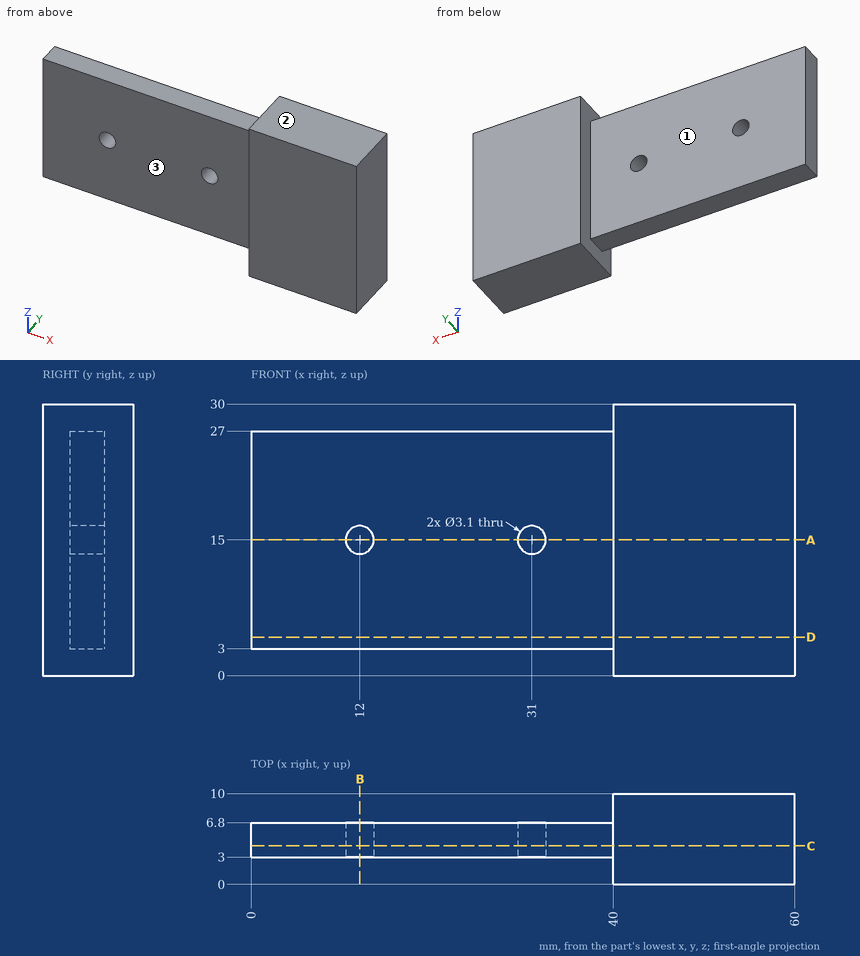
Geometry: see drawing. Coordinates: mm, zero at the bounding-box minimum. Round coordinates to 2 decimals unless told otherwise and drop trailing zeros. Write each loop counter-clockwise with the first axis right and the second up, starting at its lowest first coordinate (ties: lowest second). Pieces come first, ordered by that corner, then holes.
Item 1: Section query A-A (z = 15). Return loops of the section in (x, y), plus the area to 3 significant figures.
Item 2: Pin query (flat end, axial travel): P1, Ø1.9, axis at x = 12, z = 15, coming from the +Y side; P2, Ø3, axis at x = 21.5, z = 25.5, coming from the -Y side; P3, Ø6, axis at x = 32.5, y = 8, coming from the +Z side; P4, Ø4, axis at x = 17, y = 1.5, coming from the -Z side. Return the tip coordinate at first contact, or that it passes through.
Item 3: Material intervals for L1, parallel to X at y = 4.9, z = 15; L2, parallel to Z at x = 15, y = 5.25; L3, parallel to Y at x = 21.5, z = 21.25, sorted ascending.
Item 4: Section query B-B (x = 12). Return loops of the section in (y, z).
Item 5: Mould query, pull axis Y, two halves, no side actions, for the marked faces 1, 2 and 3. Classes: +Y half, -Y half, draft (parallel to the pull), parting line (faces both ways), or undercut.
Item 6: Section query C-C (y = 4.25). Return loops of the section in (x, z).
Item 7: Section query D-D (z = 4.25). Return loops of the section in (x, y), plus the area to 3 significant figures.
Completed:
1. outline: (0, 3) - (10.45, 3) - (10.45, 6.8) - (0, 6.8) - close; (13.55, 3) - (29.45, 3) - (29.45, 6.8) - (13.55, 6.8) - close; (32.55, 3) - (40, 3) - (40, 0) - (60, 0) - (60, 10) - (40, 10) - (40, 6.8) - (32.55, 6.8) - close
1. area: 328 mm2
2. P1: passes through
2. P2: stops at y = 3
2. P3: stops at z = 27
2. P4: stops at z = 3
3. L1: x = 0 to 10.45, 13.55 to 29.45, 32.55 to 60
3. L2: z = 3 to 27
3. L3: y = 3 to 6.8
4. outline: (3, 3) - (6.8, 3) - (6.8, 13.45) - (3, 13.45) - close; (3, 16.55) - (6.8, 16.55) - (6.8, 27) - (3, 27) - close
5. face 1: +Y half
5. face 2: draft
5. face 3: -Y half
6. outline: (0, 3) - (40, 3) - (40, 0) - (60, 0) - (60, 30) - (40, 30) - (40, 27) - (0, 27) - close; hole circle Ø3.1 at (12, 15); hole circle Ø3.1 at (31, 15)
7. outline: (0, 3) - (40, 3) - (40, 0) - (60, 0) - (60, 10) - (40, 10) - (40, 6.8) - (0, 6.8) - close
7. area: 352 mm2
